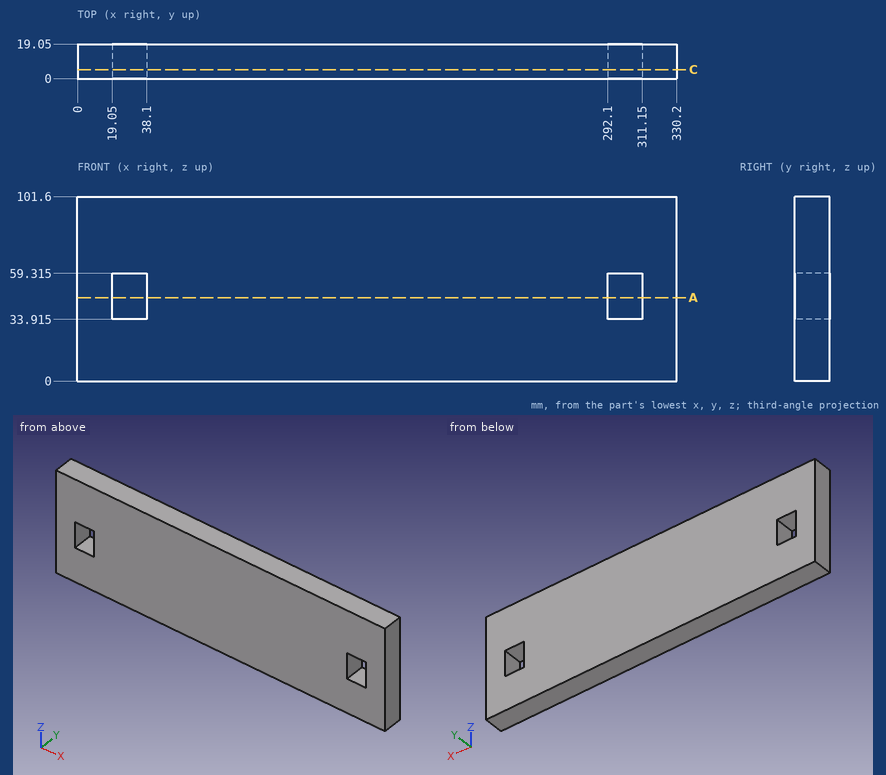
Verification items for this drawing (mm, ordinates from the low corner). Coordinates: 2 decimals unless noted, no trailing zeros. Order: outer loops, then holes, each group sorted by start corner. A loop starts at its lowest first (then second) coordinate and runs counter-clockwise, first axis right, second up. Notation, with made-up numbers: M -37,46.25 L -21,46.25 A33 cw -21,85.25 Z; hole C -33,47 d9. An arc over 180 degrees is marked long. One line per item, written item: value. Start each with the question number.
Item 1: Sectioned sample at C-C on y = 5. Give the number of separate pieces and of enclosed holes in the cut face, then the cut area to 3 significant figures.
Item 2: Sectioned sample at A-A on z = 46. Record the cut outline in (x, y).
Item 3: Thickness scan on probe 1 along X at (y, z) = (16.75, 41); probe 2 along Z at (x, y) = (34.5, 9.5) (1 decimal). Record the ranges inside material, lowest first.
Calculated:
1. separate pieces: 1
1. enclosed holes: 2
1. area: 32,600 mm^2
2. outline: M 0,0 L 19.05,0 L 19.05,19.05 L 0,19.05 Z; M 38.1,0 L 292.1,0 L 292.1,19.05 L 38.1,19.05 Z; M 311.15,0 L 330.2,0 L 330.2,19.05 L 311.15,19.05 Z
3. probe 1: 0 to 19.05, 38.1 to 292.1, 311.15 to 330.2
3. probe 2: 0 to 33.9, 59.3 to 101.6
